```python
from build123d import *

# Parameters (mm, degrees)
CROQUIS1_W            = 77.5
CROQUIS1_H            = 20.5
CROQUIS1_R            = 1.5
BRIDA_BASE1_DEPTH     = 0.5
CROQUIS2_R            = 1.5
CROQUIS2_R_2          = 2.5
CORTAR_EXTRUIR1_DEPTH = 10


# Sheet-metal steps are written as plain solids
with BuildPart() as part:
    # Croquis1 → Brida base1 (new body)
    with BuildSketch(Plane(origin=(0, 0, 0), x_dir=(1, 0, 0), z_dir=(0, 1, 0))):
        with Locations((-15.796159052, -24.916988156)):
            Rectangle(CROQUIS1_W, CROQUIS1_H)
        with Locations(Location((-50.546159052, -24.916988156, 0), (0, 0, 270))):
            Circle(CROQUIS1_R, mode=Mode.SUBTRACT)
        with Locations(Location((18.953840948, -24.916988156, 0), (0, 0, 90))):
            Circle(CROQUIS1_R, mode=Mode.SUBTRACT)
    extrude(amount=-BRIDA_BASE1_DEPTH)

    # Croquis2 → Cortar-Extruir1 (cut)
    with BuildSketch(Plane(origin=(0, 0, 0), x_dir=(-1, 0, 0), z_dir=(0, 1, 0))):
        with Locations(Location((-7.203840948, 24.916988156, 0), (0, 0, 90))):
            Circle(CROQUIS2_R)
        with Locations(Location((-7.203840948, 18.916988156, 0), (0, 0, 90))):
            Circle(CROQUIS2_R_2)
    extrude(amount=-CORTAR_EXTRUIR1_DEPTH, mode=Mode.SUBTRACT)


solid = part.part
```
For this review, take the finished solid that the model builds, in its own axes (mm). Give positions to 0.01 mm unless a question says otherwise; leave off trailing zeros. Write each loop counter-clockwise with the first axis right and the second up, starting at its lowest first coordinate (ties: lowest second). Pieces come first, ordered by that corner, then holes. Notation, with made-up numbers: M 6.5,3.25 L 50.5,3.25 A17 cw 50.5,14.25 Z; hole C 57,9.5 d7. An arc over 180 degrees is marked long. One line per item, written item: value.
1) Take a section at B-B, the plane z = 25. Write out the cut boundary in (x, y).
Results are:
outline: M -54.55,-0.5 L -52.04,-0.5 L -52.04,0 L -54.55,0 Z; M -49.05,-0.5 L 5.71,-0.5 L 5.71,0 L -49.05,0 Z; M 8.7,-0.5 L 17.46,-0.5 L 17.46,0 L 8.7,0 Z; M 20.45,-0.5 L 22.95,-0.5 L 22.95,0 L 20.45,0 Z
2) The part is to be moulded in two halves that separate along Z. For faces 1 (the flat face through (-16, -0.5, 25)), 2 (the cylindrical face through (18.503, -0.246, 23.486)), say which applies: +Z half, -Z half, draft (parallel to the pull), parting line (faces both ways), or undercut.
Results are:
face 1: draft
face 2: undercut
3) Take a section at A-A, the plane y = -0.4. Write out the cut boundary in (x, z), then the cut area to 3 significant figures.
Results are:
outline: M -54.55,14.67 L 22.95,14.67 L 22.95,35.17 L -54.55,35.17 Z; hole C -50.55,24.92 d3; hole C 7.2,18.92 d5; hole C 7.2,24.92 d3; hole C 18.95,24.92 d3
area: 1,550 mm²
4) For line 1 (X direction, y = -0.4, z = 19); line 2 (X direction, y = -0.4, z = 25.5); line 3 (X direction, y = -0.2, z = 18), list the stretches that pass through material, from the lowest coordinate up. Write a range as from..to.
Results are:
line 1: x = -54.55..4.71, 9.7..22.95
line 2: x = -54.55..-51.93, -49.16..5.82, 8.59..17.57, 20.34..22.95
line 3: x = -54.55..4.88, 9.53..22.95
